```python
from build123d import *

# Parameters (mm, degrees)
BOSS_EXTRUDE1_DEPTH = 3
BOSS_EXTRUDE2_DEPTH = 4


with BuildPart() as part:
    # Sketch1 → Boss-Extrude1 (new body)
    with BuildSketch(Plane(origin=(0, 0, 0), x_dir=(1, 0, 0), z_dir=(0, 1, 0))):
        Polygon((0, 0), (-3, 4), (0, 4), align=None)
    extrude(amount=BOSS_EXTRUDE1_DEPTH)

    # Sketch2 → Boss-Extrude2 (add)
    with BuildSketch(Plane(origin=(0, 0, -4), x_dir=(-1, 0, 0), z_dir=(0, 0, -1))):
        Polygon((0, 5), (-3, 0), (0, 0), (0, 3), align=None)
    extrude(amount=-BOSS_EXTRUDE2_DEPTH)


solid = part.part
```
Verification items for the finished model (mm, model axes). A direction names the side the tool comes from. Round coordinates to 2 decimals unless told otherwise and drop trailing zeros. Write each loop counter-clockwise with the first axis right and the second up, starting at its lowest first coordinate (ties: lowest second). Pieces come first, ordered by that corner, then holes. Notation, with made-up numbers: (75.5, 3) - (99.5, 3) arc R13 ccw to (99.5, 23) - close; hole circle Ø2 at (-6.75, 88.25). An arc over 180 degrees is marked (long way). Answer as a JSON object with one key per item and string values. Group by question number.
Q1. Go/stop test with flat-tipped pins: pin 1 Ø2 at (x, z) = (2, -2) entering from +Y; pin 2 Ø0.6 at (y, z) = (3.5, -1) entering from -X. Record where each tip stops, or that it passes through.
Q2. Section check D-D, the plane z = -3.4. Enter the section's corners in (x, y).
Q3. Section check A-A, the plane z = -1.2. Enter the section's corners in (x, y), plus the area to 3 significant figures.
Q4. Thickness scan on line 1 (Y direction, x = -0.85, z = -1.4); line 2 (Z direction, x = -2.35, y = 0.65); line 3 (X direction, y = 4.3, z = -3.35). Record the ranges inside material, lowest first.
Q5. Section check B-B, the plane y = 4.65. Enter the section's corners in (x, z), plus the area to 3 significant figures.
Q6. Tool access check on faces 1 (the flat face through (0, 4, -2)), 2 (the flat face through (1, 1, 0)). Record the directions out of +Z, -Z, +X, -X, +Y, -Y that give a thin tool (end or side, any length) a straight path to the whole face; none if there is none.
Q7. Section check C-C, the plane x = 1.7. Enter the section's corners in (y, z).
Found:
{
 "1": {"pin 1": "stops at y = 3.33", "pin 2": "stops at x = 0"},
 "2": {"outline": "(-2.55, 0) - (3, 0) - (0, 5) - (0, 3) - (-2.55, 3) - close"},
 "3": {"outline": "(-0.9, 0) - (3, 0) - (0, 5) - (0, 3) - (-0.9, 3) - close", "area": "10.2 mm^2"},
 "4": {"line 1": "y = 0 to 3", "line 2": "z = -4 to -3.13", "line 3": "x = 0 to 0.42"},
 "5": {"outline": "(0, -4) - (0.21, -4) - (0.21, 0) - (0, 0) - close", "area": "0.840 mm^2"},
 "6": {"face 1": "+Z, -Z, -X, +Y", "face 2": "+Z, +X, -X, +Y, -Y"},
 "7": {"outline": "(0, -4) - (2.17, -4) - (2.17, 0) - (0, 0) - close"}
}
